Can you work these out from the model? Positions are in its coordinate system, mm. Give positions to 0.01 mm unless a question says otherwise; leave off trailing zeros. Write each loop counter-clockwise with the first axis right and the second up, starting at its lowest first coordinate (ties: lowest second). Pieces come first, ordered by that corner, then holes.
1. Suppose I cut it at A-A (x = 163). Please give me the cut outline in (y, z), and give its area (3 significant figures).
2. Suppose I cut it at B-B (y = -49.5). Please give me the cut outline in (x, z), and give its area (3 significant figures).
3. I'm going to push flat-ended pins straight in: pin 1 (1.5 mm diameter, centred on x = -112.5, z = 2, fed in from -Y); pin 2 (2 mm diameter, centred on x = -146.5, z = 2, fed in from +Y). Where does each tip first touch, or does it pass through?
4. Suppose I cut it at C-C (z = 4). Please give me the cut outline in (x, y).
5. If I drill on probe 1 along Y at (x, z) = (-172.5, 4); probe 2 along X at (y, z) = (30, 2), over which ranges is the centre line in solid material (lowest first)?
```python
from build123d import *

# Parameters (mm, degrees)
SKETCH1_W           = 444.2968
SKETCH1_H           = 109.78515
BOSS_EXTRUDE1_DEPTH = 6.35


with BuildPart() as part:
    # Sketch1 → Boss-Extrude1 (new body)
    with BuildSketch(Plane.XY):
        Polygon((222.1484, -63.35395), (228.7016, -63.35395), (228.7016, 63.35395), (222.1484, 63.35395), (222.1484, 61.445775), (-222.1484, 61.445775), (-222.1484, 63.35395), (-228.7016, 63.35395), (-228.7016, -63.35395), (-222.1484, -63.35395), (-222.1484, -61.445775), (222.1484, -61.445775), align=None)
        Rectangle(SKETCH1_W, SKETCH1_H, mode=Mode.SUBTRACT)
    extrude(amount=BOSS_EXTRUDE1_DEPTH)


solid = part.part
```
Checks:
1. outline: (-61.45, 0) - (-54.89, 0) - (-54.89, 6.35) - (-61.45, 6.35) - close; (54.89, 0) - (61.45, 0) - (61.45, 6.35) - (54.89, 6.35) - close
1. area: 83.2 mm2
2. outline: (-228.7, 0) - (-222.15, 0) - (-222.15, 6.35) - (-228.7, 6.35) - close; (222.15, 0) - (228.7, 0) - (228.7, 6.35) - (222.15, 6.35) - close
2. area: 83.2 mm2
3. pin 1: stops at y = -61.45
3. pin 2: stops at y = 61.45
4. outline: (-228.7, -63.35) - (-222.15, -63.35) - (-222.15, -61.45) - (222.15, -61.45) - (222.15, -63.35) - (228.7, -63.35) - (228.7, 63.35) - (222.15, 63.35) - (222.15, 61.45) - (-222.15, 61.45) - (-222.15, 63.35) - (-228.7, 63.35) - close; hole (-222.15, -54.89) - (222.15, -54.89) - (222.15, 54.89) - (-222.15, 54.89) - close
5. probe 1: y = -61.45 to -54.89, 54.89 to 61.45
5. probe 2: x = -228.7 to -222.15, 222.15 to 228.7
